The listing builds one solid part. Answer for the finished solid, in the listing's coordinates (mm). Give positions to 0.01 mm unless a question says otherwise; leave off trailing zeros. Write each loop counter-clockwise with the first axis right and the second up, starting at its lowest first coordinate (ties: lowest second). Pieces come first, ordered by that corner, then holes.
Autodesk Inventor part; units mm, degrees
ref_plane "YZ Plane" through (0, 0, 0) normal (1, 0, 0) x (0, 1, 0)
ref_plane "XZ Plane" through (0, 0, 0) normal (0, 1, 0) x (-1, 0, 0)
ref_plane "XY Plane" through (0, 0, 0) normal (0, 0, 1) x (1, 0, 0)
sketch "Sketch1" plane through (0, 0, 0) normal (0, 1, 0) x (-1, 0, 0)
  line L0 (0, 0) -> (101.6, 0)
  line L1 (0, -12.7) -> (44.45, -12.7)
  line L2 (44.45, -12.7) -> (76.2, -12.7)
  line L3 (44.45, 0) -> (76.2, -6.35)
  line L4 (76.2, -6.35) -> (101.6, -6.35)
  line L5 (76.2, -12.7) -> (101.6, -12.7)
  line L6 (0, -12.7) -> (0, 0)
  line L7 (101.6, -12.7) -> (101.6, -6.35)
  point P0 (101.6, -6.35)
  dimension "d5" = 44.45
  dimension "d6" = 12.7
  dimension "d7" = 44.45
  dimension "d16" = 6.35
  dimension "d55" = 6.35
  dimension "d58" = 31.75
  dimension "d59" = 101.6
extrude "Extrusion2" add sketch "Sketch1" along normal blind 6.35
sketch "Sketch5" plane through (0, 6.35, 0) normal (0, 1, 0) x (1, 0, 0)
  line L0 (-44.45, 0) -> (0, 0)
  line L1 (0, 0) -> (0, 12.7)
  line L2 (0, 12.7) -> (-101.6, 12.7)
  line L3 (-101.6, 12.7) -> (-101.6, 6.35)
  line L4 (-101.6, 6.35) -> (-76.2, 6.35)
  line L5 (-76.2, 6.35) -> (-44.45, 0)
  point P0 (-6.35, 6.35)
  point P1 (-34.925, 6.35)
  dimension "d60" = 6.35
  dimension "d61" = 6.35
  dimension "d62" = 6.35
  dimension "d63" = 28.575
  dimension "d64" = 12.7
hole "Hole4" at (-6.35, 6.35, -6.35) at (-34.925, 6.35, -6.35) direction (0, -1, 0) diameter 8.382 depth 25.4 tip angle 118
sketch "Sketch6" plane through (-101.6, 0, -6.35) normal (0, 0, 1) x (1, 0, 0)
  line L0 (25.4, 0) -> (0, 0)
  line L1 (25.4, 0) -> (25.4, 6.35)
  line L2 (0, 6.35) -> (25.4, 6.35)
  line L3 (0, 0) -> (0, 6.35)
  point P0 (101.6, 0)
  point P1 (3.175, 3.175)
  point P2 (22.225, 3.175)
  dimension "d72" = 6.35
  dimension "d73" = 3.175
  dimension "d74" = 3.175
  dimension "d75" = 19.05
  dimension "d76" = 3.175
hole "Hole5" at (-98.425, 3.175, -6.35) at (-79.375, 3.175, -6.35) direction (0, 0, -1) diameter 2.6416 depth 10.9728 tip angle 118
equation "\"d5\" = d10"
equation "\"d7\" = d5"
properties part number "WheelSuspensionFork" material "Aluminum 6061"
Item 1: A cutting plane is placed at B-B, the plane y = 3.25. Give the vertices of the cut face in (x, z) (3 decimals), plus the area to 3 significant figures.
Conclusion:
outline: (-101.6, -12.7) - (-99.744, -12.7) - (-99.744, -6.35) - (-101.6, -6.35) - close; (-97.106, -12.7) - (-80.694, -12.7) - (-80.694, -6.35) - (-97.106, -6.35) - close; (-78.056, -12.7) - (0, -12.7) - (0, 0) - (-44.45, 0) - (-76.2, -6.35) - (-78.056, -6.35) - close; hole circle Ø8.382 at (-34.925, -6.35); hole circle Ø8.382 at (-6.35, -6.35)
area: 884 mm2
Item 2: A cutting plane is placed at A-A, the plane x = -6.35. Give the vertices of the cut face in (y, z), plus the area to 3 significant figures.
Conclusion:
outline: (0, -12.7) - (6.35, -12.7) - (6.35, -10.54) - (0, -10.54) - close; (0, -2.16) - (6.35, -2.16) - (6.35, 0) - (0, 0) - close
area: 27.4 mm2
Item 3: A cutting plane is placed at C-C, the plane z = -7.75. Give the vertices of the cut face in (x, y) (3 decimals), plus the area to 3 significant figures.
Conclusion:
outline: (-101.6, 0) - (-38.875, 0) - (-38.875, 6.35) - (-101.6, 6.35) - close; (-30.975, 0) - (-10.3, 0) - (-10.3, 6.35) - (-30.975, 6.35) - close; (-2.4, 0) - (0, 0) - (0, 6.35) - (-2.4, 6.35) - close; hole circle Ø2.642 at (-98.425, 3.175); hole circle Ø2.642 at (-79.375, 3.175)
area: 534 mm2
Item 4: Determine the mould class of faces 1 (the face through (-89, 3, -6.35)), 2 (the face through (0, 3, -6)), 3 (the face through (-30.834, 3.131, -7.259)) for opening direction Z: pulls with the +Z half, pulls with the -Z half, needs draft (parallel to the pull), parting line crosses it, or undercut.
Conclusion:
face 1: pulls with the +Z half
face 2: needs draft
face 3: undercut
Item 5: Consider probe 1 along X at (y, z) = (1.25, -9.5); probe 2 along X at (y, z) = (5.5, -7); probe 3 along Z at (x, y) = (-86, 3). Determine where each line is inside the solid, lowest interval first.
Conclusion:
probe 1: x = -101.6 to -37.69, -32.16 to -9.11, -3.59 to 0
probe 2: x = -101.6 to -39.07, -30.78 to -10.49, -2.21 to 0
probe 3: z = -12.7 to -6.35
Item 6: A cutting plane is placed at D-D, the plane x = -58. Give the vertices of the cut face in (y, z), plus the area to 3 significant figures.
Conclusion:
outline: (0, -12.7) - (6.35, -12.7) - (6.35, -2.71) - (0, -2.71) - close
area: 63.4 mm2
